Read the model definition and answer for the solid it produces. Units are mm, in the model's axes. A direction names the side the tool comes from. Coordinates: 2 decimals unless noted, no trailing zeros. Loops run counter-clockwise (first coordinate to the right, second up) from the corner with the lowest first, then second, coordinate; pieces in that order, holes last. Notation, with made-up numbers: (58.5, 7) -> (70.5, 7) arc R21 ccw to (70.5, 33) -> close; hole circle Ø5 at (61, -24). An arc over 180 degrees is marked (long way). Answer in a Markdown table with one row per item.
```python
from build123d import *

# Parameters (mm, degrees)
SKETCH1_W           = 40.005
SKETCH1_H           = 28.575
BOSS_EXTRUDE1_DEPTH = 2.54
SKETCH2_R           = 1.5875
CUT_EXTRUDE1_DEPTH  = 25.712026677
SKETCH3_R           = 14.2875
BOSS_EXTRUDE2_DEPTH = 6.35
SKETCH4_R           = 8.4455
BOSS_EXTRUDE3_DEPTH = 3.429
FILLET1_R           = 0.254
SKETCH5_W           = 6.003121546
SKETCH5_H           = 5.08
BOSS_EXTRUDE4_DEPTH = 3.175
BOSS_EXTRUDE5_DEPTH = 6.35
BOSS_EXTRUDE6_DEPTH = 1.27
FILLET2_R           = 1.016
CUT_EXTRUDE2_DEPTH  = 5.08


with BuildPart() as part:
    # Sketch1 → Boss-Extrude1 (new body)
    with BuildSketch(Plane(origin=(0, 0, 0), x_dir=(1, 0, 0), z_dir=(0, 1, 0))):
        Rectangle(SKETCH1_W, SKETCH1_H)
    extrude(amount=BOSS_EXTRUDE1_DEPTH)

    # Sketch2 → Cut-Extrude1 (cut, through all)
    with BuildSketch(Plane(origin=(0, 0, 0), x_dir=(1, 0, 0), z_dir=(0, 1, 0))):
        with Locations(Location((-16.51, 11.1125, 0), (0, 0, 270))):
            Circle(SKETCH2_R)
        with Locations(Location((16.51, 11.1125, 0), (0, 0, 270))):
            Circle(SKETCH2_R)
        with Locations(Location((16.51, -11.1125, 0), (0, 0, 270))):
            Circle(SKETCH2_R)
        with Locations(Location((-16.51, -11.1125, 0), (0, 0, 270))):
            Circle(SKETCH2_R)
    extrude(amount=CUT_EXTRUDE1_DEPTH, mode=Mode.SUBTRACT)

    # Sketch3 → Boss-Extrude2 (add)
    with BuildSketch(Plane(origin=(0, 2.54, 0), x_dir=(1, 0, 0), z_dir=(0, 1, 0))):
        with Locations(Location((0, 0, 0), (0, 0, 270))):
            Circle(SKETCH3_R)
    extrude(amount=BOSS_EXTRUDE2_DEPTH)

    # Sketch4 → Boss-Extrude3 (add)
    with BuildSketch(Plane(origin=(0, 8.89, 0), x_dir=(1, 0, 0), z_dir=(0, 1, 0))):
        with Locations(Location((0, 0, 0), (0, 0, 270))):
            Circle(SKETCH4_R)
    extrude(amount=BOSS_EXTRUDE3_DEPTH)

    # Fillet1
    fillet1_edges = [part.edges().sort_by_distance(p)[0] for p in [
        (0, 12.319, -8.4455),
    ]]
    fillet(fillet1_edges, radius=FILLET1_R)

    # Sketch5 → Boss-Extrude4 (add)
    with BuildSketch(Plane(origin=(0, 2.54, 0), x_dir=(1, 0, 0), z_dir=(0, 1, 0))):
        with Locations((-16.138348766, 0)):
            Rectangle(SKETCH5_W, SKETCH5_H)
    extrude(amount=BOSS_EXTRUDE4_DEPTH)

    # Sketch6 → Boss-Extrude5 (add)
    with BuildSketch(Plane(origin=(0, 2.54, 0), x_dir=(1, 0, 0), z_dir=(0, 1, 0))):
        with BuildLine():
            Line((11.184835996, -8.89), (17.918367846, -8.89))
            ThreePointArc((17.918367846, -8.89), (20.0025, 0), (17.918367846, 8.89))
            Line((17.918367846, 8.89), (11.184835996, 8.89))
            ThreePointArc((11.184835996, 8.89), (14.2875, 0), (11.184835996, -8.89))
        make_face()
    extrude(amount=BOSS_EXTRUDE5_DEPTH)

    # Sketch7 → Boss-Extrude6 (add, symmetric)
    with BuildSketch(Plane(origin=(0, 8.89, 0), x_dir=(1, 0, 0), z_dir=(0, 1, 0))):
        with BuildLine():
            Line((13.281601921, 7.62), (13.281601921, 10.16))
            ThreePointArc((13.281601921, 10.16), (14.551601921, 11.43), (15.821601921, 10.16))
            Line((15.821601921, 10.16), (15.821601921, 7.62))
            ThreePointArc((15.821601921, 7.62), (14.551601921, 6.35), (13.281601921, 7.62))
        make_face()
        with BuildLine():
            Line((13.281601921, -7.62), (13.281601921, -10.16))
            ThreePointArc((13.281601921, -10.16), (14.551601921, -11.43), (15.821601921, -10.16))
            Line((15.821601921, -10.16), (15.821601921, -7.62))
            ThreePointArc((15.821601921, -7.62), (14.551601921, -6.35), (13.281601921, -7.62))
        make_face()
    extrude(amount=BOSS_EXTRUDE6_DEPTH, both=True)

    # Fillet2
    fillet2_edges = [part.edges().sort_by_distance(p)[0] for p in [
        (13.281601921, 7.62, 9.525),
        (14.551601921, 7.62, 11.43),
        (15.821601921, 7.62, 9.525),
        (14.551601921, 10.16, 6.35),
        (13.281601921, 10.16, 8.89),
        (14.551601921, 10.16, 11.43),
        (15.821601921, 10.16, 8.89),
        (15.821601921, 7.62, -9.525),
        (14.551601921, 7.62, -11.43),
        (13.281601921, 7.62, -9.525),
        (14.551601921, 10.16, -6.35),
        (15.821601921, 10.16, -8.89),
        (14.551601921, 10.16, -11.43),
        (13.281601921, 10.16, -8.89),
    ]]
    fillet(fillet2_edges, radius=FILLET2_R)

    # Sketch9 → Cut-Extrude2 (cut)
    with BuildSketch(Plane(origin=(0, 2.54, 0), x_dir=(1, 0, 0), z_dir=(0, 1, 0))):
        with BuildLine():
            Line((0, 14.2875), (31.753560491, 14.2875))
            Line((31.753560491, 14.2875), (31.753560491, 3.4925))
            Line((31.753560491, 3.4925), (13.854064386, 3.4925))
            ThreePointArc((13.854064386, 3.4925), (8.781616096, 11.270131987), (0, 14.2875))
        make_face()
        with BuildLine():
            Line((13.854064386, -3.4925), (31.753560491, -3.4925))
            Line((31.753560491, -3.4925), (31.753560491, -14.2875))
            Line((31.753560491, -14.2875), (0, -14.2875))
            ThreePointArc((0, -14.2875), (8.781616096, -11.270131987), (13.854064386, -3.4925))
        make_face()
    extrude(amount=CUT_EXTRUDE2_DEPTH, mode=Mode.SUBTRACT)


solid = part.part
```
1. A tool of negligible diameter and unlimited length cuts with its end or side. For faces 1 (the flat face through (17, 5, -3.492)), 2 (the cylindrical face through (2.537, 10.455, 8.056)), 3 (the flat face through (-17, 4, -2.54)), 4 (the cylindrical face through (20.002, 6.376, 0.129)), 5 (the flat face through (17, 5, 3.492)), from which of +Z, -Z, +X, -X, +Y, -Y can it reach the whole face along a straight path? Write none if from no direction.
A:
| item | result |
|---|---|
| face 1 | -Z, +X |
| face 2 | +Y |
| face 3 | -Z, -X, +Y |
| face 4 | +X, +Y |
| face 5 | +Z, +X |
2. Given pin 1 Ø0.6 at (x, z) = (14.5, -8.5) entering from +Y; pin 2 Ø1.6 at (x, y) = (-15.5, 4.5) entering from +Z; pin 3 Ø1.9 at (x, z) = (-16.51, -11.11) entering from -Y; pin 4 Ø3.5 at (x, z) = (16.51, 11.11) entering from +Y, each flat-ended and moving along its own axis, determine where each tip first touches the part or whether it passes through.
A:
| item | result |
|---|---|
| pin 1 | stops at y = 10.16 |
| pin 2 | stops at z = 2.54 |
| pin 3 | passes through |
| pin 4 | stops at y = 10.15 |
3. A cutting plane is placed at A-A on x = 16.51. Give the vertices of the cut face in (y, z) (1 decimal), and give its area (3 significant figures).
A:
| item | result |
|---|---|
| outline | (0, -14.3) -> (2.5, -14.3) -> (2.5, -12.7) -> (0, -12.7) -> close; (0, -9.5) -> (2.5, -9.5) -> (2.5, -3.5) -> (7.6, -3.5) -> (7.6, -8.9) -> (8.9, -8.9) -> (8.9, 8.9) -> (7.6, 8.9) -> (7.6, 3.5) -> (2.5, 3.5) -> (2.5, 9.5) -> (0, 9.5) -> close; (0, 12.7) -> (2.5, 12.7) -> (2.5, 14.3) -> (0, 14.3) -> close |
| area | 115 mm2 |
4. A cutting plane is placed at C-C on x = -16.51. Give the vertices of the cut face in (y, z) (1 decimal).
A:
| item | result |
|---|---|
| outline | (0, -14.3) -> (2.5, -14.3) -> (2.5, -12.7) -> (0, -12.7) -> close; (0, -9.5) -> (2.5, -9.5) -> (2.5, -2.5) -> (5.7, -2.5) -> (5.7, 2.5) -> (2.5, 2.5) -> (2.5, 9.5) -> (0, 9.5) -> close; (0, 12.7) -> (2.5, 12.7) -> (2.5, 14.3) -> (0, 14.3) -> close |
5. Find the intervals of material crossed by probe 1 along X at (y, z) = (1.75, -11); probe 2 along Z at (x, y) = (-16.51, 0.75) (1 decimal); probe 3 along X at (y, z) = (1, 12), in increasing order.
A:
| item | result |
|---|---|
| probe 1 | x = -20 to -18.09, -14.93 to 14.93, 18.09 to 20 |
| probe 2 | z = -14.3 to -12.7, -9.5 to 9.5, 12.7 to 14.3 |
| probe 3 | x = -20 to -17.83, -15.19 to 15.19, 17.83 to 20 |
6. A cutting plane is placed at B-B on y = 2. Give the vertices of the cut face in (x, z) (1 decimal), and give its area (3 significant figures).
A:
| item | result |
|---|---|
| outline | (-20, -14.3) -> (20, -14.3) -> (20, 14.3) -> (-20, 14.3) -> close; hole circle Ø3.2 at (-16.5, -11.1); hole circle Ø3.2 at (-16.5, 11.1); hole circle Ø3.2 at (16.5, -11.1); hole circle Ø3.2 at (16.5, 11.1) |
| area | 1,110 mm2 |
7. A cutting plane is placed at D-D on y = 11.25. Give the vertices of the cut face in (x, z).
A:
| item | result |
|---|---|
| outline | circle Ø16.89 at (0, 0) |
8. The mould has two halves that part along X. Classify faces 6 (the flat face through (20.002, 1, 0)), 7 (the cylindrical face through (13.571, 9.854, 8.908)), 8 (the cylindrical face through (16.99, 1.25, -9.6)), 9 (the flat face through (17, 8, 8.89)): pulls with the +X half, pulls with the -X half, needs draft (parallel to the pull), parting line crosses it, or undercut.
A:
| item | result |
|---|---|
| face 6 | pulls with the +X half |
| face 7 | undercut |
| face 8 | undercut |
| face 9 | needs draft |
